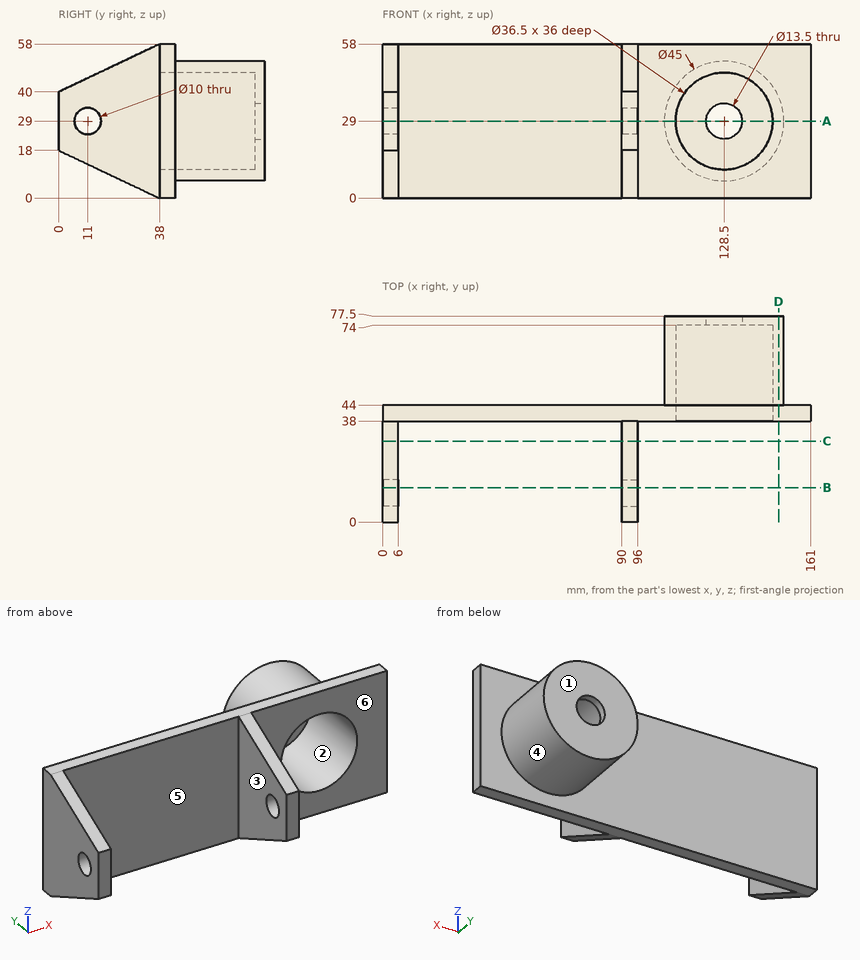
Input: dimensioned drawing with shaded views. Units: mm. Origin: part minimum x, y, z. A direction names the side the tool comes from. Round coordinates to 2 decimals unless told otherwise and drop trailing zeros. Loops run counter-clockwise (first coordinate to the right, second up) from the corner with the lowest first, then second, coordinate; pieces in that order, holes last.
1) Pin query (flat end, axial travel): pin 1 (19 mm diameter, centred on y = 22, z = 31, fed in from +X); pin 2 (4 mm diameter, centred on y = 69, z = 24, fed in from +X); pin 3 (11.5 mm diameter, centred on y = 11, z = 29, fed in from -X); pin 4 (1 mm diameter, centred on x = 90, z = 10.5, fed in from +Y). Return the tip coordinate at first contact, or that it passes through.
Ans:
pin 1: stops at x = 96
pin 2: stops at x = 150.8
pin 3: stops at x = 0
pin 4: stops at y = 44
2) Material intervals for line 1 (X direction, y = 36, z = 3); line 2 (Z direction, x = 128.5, y = 75.85); line 3 (Y direction, x = 94.25, z = 29), sorted ascending.
Ans:
line 1: x = 0 to 6, 90 to 96
line 2: z = 6.5 to 22.25, 35.75 to 51.5
line 3: y = 0 to 6, 16 to 44
3) Set-up query: the marked faces 1, 2 and 3. Return all of +Z, -Z, +X, -X, +Y, -Y with unobstructed straight access to the full face (end or side cutting, diameter ignored); none if empty.
Ans:
face 1: +Z, -Z, +X, -X, +Y
face 2: -Y
face 3: +Z, -Z, -Y
4) Section query D-D on x = 149. Return the cut outline in (y, z), plus the area to 3 significant figures.
Ans:
outline: (38, 0) - (44, 0) - (44, 19.73) - (77.5, 19.73) - (77.5, 38.27) - (44, 38.27) - (44, 58) - (38, 58) - close
area: 969 mm2
5) Pull-direction query (X, two-part tool) for the marked faces 4, 5 and 6; classes: released by +X, released by -X, zero draft, split by the parting line, or undercut.
Ans:
face 4: split by the parting line
face 5: undercut
face 6: zero draft
6) Section query B-B on y = 13. Return the cut outline in (x, z).
Ans:
outline: (0, 11.84) - (6, 11.84) - (6, 24.42) - (0, 24.42) - close; (0, 33.58) - (6, 33.58) - (6, 46.16) - (0, 46.16) - close; (90, 11.84) - (96, 11.84) - (96, 24.42) - (90, 24.42) - close; (90, 33.58) - (96, 33.58) - (96, 46.16) - (90, 46.16) - close
7) Section query A-A on z = 29. Count the separate pieces of the cut face and the enclosed holes in it, plus the area to 3 significant figures.
Ans:
separate pieces: 4
enclosed holes: 0
area: 1,450 mm2
8) Section query C-C on y = 30.5. Return the cut outline in (x, z).
Ans:
outline: (0, 3.55) - (6, 3.55) - (6, 54.45) - (0, 54.45) - close; (90, 3.55) - (96, 3.55) - (96, 54.45) - (90, 54.45) - close
